Source: CAD feature listing. Evaluate the final solid. Frame: model axes, mm. Face numbers are marked on the shaded views. Coordinates: 2 decimals unless noted, no trailing zeros. Write each loop counter-clockwise with the first axis right and the second up, starting at its lowest first coordinate (ties: lowest second). Pieces come first, ordered by that corner, then holes. Notation, with made-up numbers: (39.25, -8.75) -> (62.25, -8.75) arc R17 cw to (62.25, 19.25) -> close; hole circle Ø2 at (53.5, -21). An arc over 180 degrees is marked (long way). Write item = value, one per line.
from build123d import *

# Parameters (mm, degrees)
SKETCH1_W           = 96
SKETCH1_H           = 96
BOSS_EXTRUDE1_DEPTH = 2
SKETCH2_W           = 96
SKETCH2_H           = 96
BOSS_EXTRUDE2_DEPTH = 5
SKETCH3_W           = 6.5
SKETCH3_H           = 6.5
BOSS_EXTRUDE3_DEPTH = 6.5
SKETCH5_R           = 15
CUT_EXTRUDE1_DEPTH  = 10


with BuildPart() as part:
    # Sketch1 → Boss-Extrude1 (new body)
    with BuildSketch(Plane.XY):
        Rectangle(SKETCH1_W, SKETCH1_H)
    extrude(amount=BOSS_EXTRUDE1_DEPTH)

    # Sketch2 → Boss-Extrude2 (add)
    with BuildSketch(Plane.XY.offset(2)):
        Rectangle(SKETCH2_W, SKETCH2_H)
        with BuildLine():
            Line((37, -42), (-37, -42))
            ThreePointArc((-37, -42), (-40.535533906, -40.535533906), (-42, -37))
            Line((-42, -37), (-42, 37))
            ThreePointArc((-42, 37), (-40.535533906, 40.535533906), (-37, 42))
            Line((-37, 42), (37, 42))
            ThreePointArc((37, 42), (40.535533906, 40.535533906), (42, 37))
            Line((42, 37), (42, -37))
            ThreePointArc((42, -37), (40.535533906, -40.535533906), (37, -42))
        make_face(mode=Mode.SUBTRACT)
    extrude(amount=BOSS_EXTRUDE2_DEPTH)

    # Sketch3 → Boss-Extrude3 (add)
    with BuildSketch(Plane(origin=(0, 0, 0), x_dir=(-1, 0, 0), z_dir=(0, 0, -1))):
        with Locations((-44.75, 44.75)):
            Rectangle(SKETCH3_W, SKETCH3_H)
        with Locations((44.75, 44.75)):
            Rectangle(SKETCH3_W, SKETCH3_H)
        with Locations((-44.75, -44.75)):
            Rectangle(SKETCH3_W, SKETCH3_H)
        with Locations((44.75, -44.75)):
            Rectangle(SKETCH3_W, SKETCH3_H)
    extrude(amount=BOSS_EXTRUDE3_DEPTH)

    # Sketch5 → Cut-Extrude1 (cut)
    with BuildSketch(Plane(origin=(0, 0, 0), x_dir=(-1, 0, 0), z_dir=(0, 0, -1))):
        Circle(SKETCH5_R)
    extrude(amount=-CUT_EXTRUDE1_DEPTH, mode=Mode.SUBTRACT)


solid = part.part
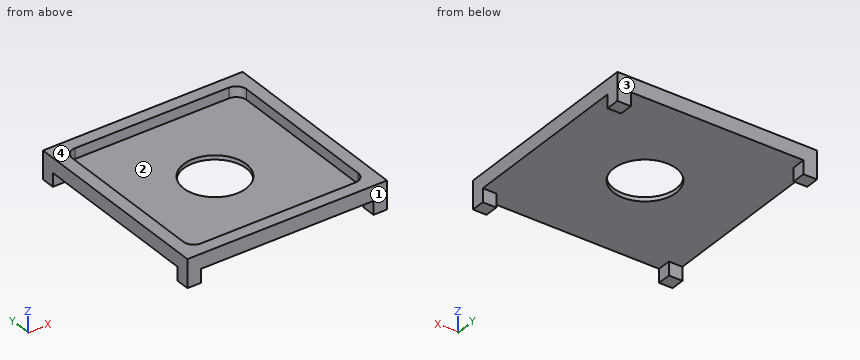
1) Pull-direction query (Y, two-part tool) for the marked faces 1, 2, 3 and 4; classes: +Y half, -Y half, draft (parallel to the pull), parting line (faces both ways), or undercut.
Answer block:
face_1 = -Y half
face_2 = undercut
face_3 = +Y half
face_4 = draft
2) Cut plane A-A, the plane x = 0. Output: boundary loops of the cut face in (y, z), and give its area (3 significant figures).
Answer block:
outline = (-48, 0) -> (-15, 0) -> (-15, 2) -> (-42, 2) -> (-42, 7) -> (-48, 7) -> close; (15, 0) -> (48, 0) -> (48, 7) -> (42, 7) -> (42, 2) -> (15, 2) -> close
area = 192 mm2
3) Cut plane B-B, the plane z = 4.25. Output: boundary loops of the cut face in (x, y), and give its area (3 significant figures).
Answer block:
outline = (-48, -48) -> (48, -48) -> (48, 48) -> (-48, 48) -> close; hole (-42, -37) arc R5 ccw to (-37, -42) -> (37, -42) arc R5 ccw to (42, -37) -> (42, 37) arc R5 ccw to (37, 42) -> (-37, 42) arc R5 ccw to (-42, 37) -> close
area = 2,180 mm2
4) First-contact query: pin 1 Ø4 at (x, y) = (-16.5, -11.5) entering from -Z; pin 2 Ø5 at (x, y) = (-32, 29.5) entering from +Z. Flat tips, straight axial feed; report the tip coordinate or a pass-through.
Answer block:
pin_1 = 0
pin_2 = 2
5) Material intervals for probe 1 along X at (y, z) = (-24.5, 5.25); probe 2 along X at (y, z) = (-42.5, -3.75); probe 3 along Y at (x, z) = (0, 0.6), sorted ascending. Write a range as [from, to].
Answer block:
probe_1 = [-48, -42], [42, 48]
probe_2 = [-48, -41.5], [41.5, 48]
probe_3 = [-48, -15], [15, 48]
6) Cut plane C-C, the plane y = -29.5. Output: boundary loops of the cut face in (x, z), and give its area (3 significant figures).
Answer block:
outline = (-48, 0) -> (48, 0) -> (48, 7) -> (42, 7) -> (42, 2) -> (-42, 2) -> (-42, 7) -> (-48, 7) -> close
area = 252 mm2
